```python
from build123d import *

# Parameters (mm, degrees)
EXTRUDE_1_DEPTH          = 3
SKETCH_13_W              = 40
SKETCH_13_H              = 2
EXTRUDE_3_DEPTH          = 15
EXTRUDE_4_DEPTH          = 20
EXTRUDE_4_DEPTH_BACK     = 20
CUT_EXTRUDE_6_DEPTH      = 18.5
CUT_EXTRUDE_6_DEPTH_BACK = 18.5
CUT_EXTRUDE_7_REACH      = 114.258
SKETCH_16_R              = 1.8
SKETCH_16_R_2            = 3.5


with BuildPart() as part:
    # 草图2 → 凸台-拉伸1 (new body)
    with BuildSketch(Plane.XY):
        with BuildLine():
            Line((0, 0), (63, 0))
            Line((63, 0), (63, 69))
            ThreePointArc((63, 69), (59.939265863, 76.389265863), (52.55, 79.45))
            Line((52.55, 79.45), (10.45, 79.45))
            ThreePointArc((10.45, 79.45), (3.060734137, 76.389265863), (0, 69))
            Line((0, 69), (0, 0))
        make_face()
    extrude(amount=EXTRUDE_1_DEPTH)

    # 草图13 → 凸台-拉伸3 (add)
    with BuildSketch(Plane(origin=(0, 0, 3), x_dir=(-1, 0, 0), z_dir=(0, 0, -1))):
        with Locations((-31.5, 80.45)):
            Rectangle(SKETCH_13_W, SKETCH_13_H)
    extrude(amount=EXTRUDE_3_DEPTH)

    # 草图14 → 凸台-拉伸4 (add, two sides: drawn at the far end of the back side and taken through both)
    with BuildSketch(Plane.ZY.offset(-31.5).offset(-EXTRUDE_4_DEPTH_BACK)):
        with BuildLine():
            ThreePointArc((3, 79.45), (10.588190451, 78.450995775), (16.660254038, 83.110254038))
            ThreePointArc((16.660254038, 83.110254038), (17.659258263, 85.522063587), (18, 88.110254038))
            ThreePointArc((18, 88.110254038), (11.686285655, 97.406021788), (0.717740386, 94.9636251))
            ThreePointArc((0.717740386, 94.9636251), (-1.999142036, 88.241244641), (0.540709407, 81.45))
            Line((0.540709407, 81.45), (3, 81.45))
            Line((3, 81.45), (3, 79.45))
        make_face()
        with BuildLine():
            ThreePointArc((0.540709407, 81.45), (1.690603791, 80.351934666), (3, 79.45))
            Line((3, 79.45), (3, 81.45))
            Line((3, 81.45), (0.540709407, 81.45))
        make_face()
        with BuildLine():
            ThreePointArc((0.540709407, 81.45), (-1.999142036, 88.241244641), (0.717740386, 94.9636251))
            Line((0.717740386, 94.9636251), (-12, 81.45))
            Line((-12, 81.45), (0.540709407, 81.45))
        make_face()
        with BuildLine():
            Line((3, 59.45), (16.660254038, 83.110254038))
            ThreePointArc((16.660254038, 83.110254038), (10.588190451, 78.450995775), (3, 79.45))
            Line((3, 79.45), (3, 59.45))
        make_face()
    extrude(amount=EXTRUDE_4_DEPTH + EXTRUDE_4_DEPTH_BACK)

    # 草图15 → 切除-拉伸6 (cut, two sides: drawn at the far end of the back side and taken through both)
    with BuildSketch(Plane.ZY.offset(-31.5).offset(-CUT_EXTRUDE_6_DEPTH_BACK)):
        with BuildLine():
            Line((0, 59.45), (3, 59.45))
            Line((3, 59.45), (16.660254038, 83.110254038))
            ThreePointArc((16.660254038, 83.110254038), (13.96660025, 96.13519525), (0.717740386, 94.9636251))
            Line((0.717740386, 94.9636251), (-12, 81.45))
            Line((-12, 81.45), (0, 81.45))
            Line((0, 81.45), (0, 59.45))
        make_face()
    extrude(amount=CUT_EXTRUDE_6_DEPTH + CUT_EXTRUDE_6_DEPTH_BACK, mode=Mode.SUBTRACT)

    # 切除-拉伸7: up to this face of the body (flat: up to its plane)
    cut_extrude_7_end = Plane(part.part.faces().sort_by_distance((51.5, 84.002247989, 5.535309017))[0])
    # 草图16 → 切除-拉伸7 (cut, up to the picked face)
    with BuildSketch(Plane.ZY.offset(-11.5), mode=Mode.PRIVATE) as cut_extrude_7_sk1:
        with Locations(Location((8, 95.110254038, 0), (0, 0, 270))):
            Circle(SKETCH_16_R)
    cut_extrude_7_tool1 = split(extrude(cut_extrude_7_sk1.sketch, amount=-CUT_EXTRUDE_7_REACH, mode=Mode.PRIVATE), bisect_by=cut_extrude_7_end, keep=Keep.BOTH, mode=Mode.PRIVATE)
    # 草图16 → 切除-拉伸7 (cut, up to the picked face)
    with BuildSketch(Plane.ZY.offset(-11.5), mode=Mode.PRIVATE) as cut_extrude_7_sk2:
        with Locations(Location((15, 88.110254038, 0), (0, 0, 270))):
            Circle(SKETCH_16_R)
    cut_extrude_7_tool2 = split(extrude(cut_extrude_7_sk2.sketch, amount=-CUT_EXTRUDE_7_REACH, mode=Mode.PRIVATE), bisect_by=cut_extrude_7_end, keep=Keep.BOTH, mode=Mode.PRIVATE)
    # 草图16 → 切除-拉伸7 (cut, up to the picked face)
    with BuildSketch(Plane.ZY.offset(-11.5), mode=Mode.PRIVATE) as cut_extrude_7_sk3:
        with Locations(Location((8, 81.110254038, 0), (0, 0, 270))):
            Circle(SKETCH_16_R)
    cut_extrude_7_tool3 = split(extrude(cut_extrude_7_sk3.sketch, amount=-CUT_EXTRUDE_7_REACH, mode=Mode.PRIVATE), bisect_by=cut_extrude_7_end, keep=Keep.BOTH, mode=Mode.PRIVATE)
    # 草图16 → 切除-拉伸7 (cut, up to the picked face)
    with BuildSketch(Plane.ZY.offset(-11.5), mode=Mode.PRIVATE) as cut_extrude_7_sk4:
        with Locations(Location((1, 88.110254038, 0), (0, 0, 270))):
            Circle(SKETCH_16_R)
    cut_extrude_7_tool4 = split(extrude(cut_extrude_7_sk4.sketch, amount=-CUT_EXTRUDE_7_REACH, mode=Mode.PRIVATE), bisect_by=cut_extrude_7_end, keep=Keep.BOTH, mode=Mode.PRIVATE)
    # 草图16 → 切除-拉伸7 (cut, up to the picked face)
    with BuildSketch(Plane.ZY.offset(-11.5), mode=Mode.PRIVATE) as cut_extrude_7_sk5:
        with Locations(Location((8, 88.110254038, 0), (0, 0, 270))):
            Circle(SKETCH_16_R_2)
    cut_extrude_7_tool5 = split(extrude(cut_extrude_7_sk5.sketch, amount=-CUT_EXTRUDE_7_REACH, mode=Mode.PRIVATE), bisect_by=cut_extrude_7_end, keep=Keep.BOTH, mode=Mode.PRIVATE)
    add(cut_extrude_7_tool1.solids().sort_by(Axis((11.5, 95.110254, 8), (1, 0, 0)))[0], mode=Mode.SUBTRACT)
    add(cut_extrude_7_tool2.solids().sort_by(Axis((11.5, 88.110254, 15), (1, 0, 0)))[0], mode=Mode.SUBTRACT)
    add(cut_extrude_7_tool3.solids().sort_by(Axis((11.5, 81.110254, 8), (1, 0, 0)))[0], mode=Mode.SUBTRACT)
    add(cut_extrude_7_tool4.solids().sort_by(Axis((11.5, 88.110254, 1), (1, 0, 0)))[0], mode=Mode.SUBTRACT)
    add(cut_extrude_7_tool5.solids().sort_by(Axis((11.5, 88.110254, 8), (1, 0, 0)))[0], mode=Mode.SUBTRACT)


solid = part.part
```
Part model, mm, in its own coordinate system. A direction names the side the tool comes from. Give positions to 0.01 mm unless a question says otherwise; leave off trailing zeros. Order: outer loops, then holes, each group sorted by start corner. A loop starts at its lowest first (then second) coordinate and runs counter-clockwise, first axis right, second up. Notation, with made-up numbers: M 8,-27 L 20,-27 A22 cw 20,-20 Z; hole C 40.25,-29.75 d10. An arc over 180 degrees is marked long. Use a Markdown table: item, result. Add a question column.
(1) Saw through at D-D, the plane z = 15. Give the cut face in (x, y), and give its area (3 significant figures).
(2) Drop flat-ended pins along their axis: P1, Ø4, axis at y = 81.11, z = 8, coming from the -X side; P2, Ø15, axis at y = 79.5, z = -3, coming from the -X side; P3, Ø1.6, axis at x = 37.5, y = 80, coming from the +Z side. Give the stop position or say it passes through.
(3) Mould opens along Y. For faces 4 (the face through (12.24, 86.448, 0.311)), 5 (the face through (63, 34, 1)), 6 (the face through (50.74, 93.448, 7.311)), 7 (the face through (50.76, 71.11, 9.73)) say: +Y half, -Y half, draft (parallel to the pull), parting line (faces both ways), or undercut.
(4) Probe line 1 along X through (y, z) = (70, 4.5); line 2 along Y through (x, z) = (18, -3.5); line 3 along Z through (x, y) = (56.5, 20.5). List the from-to ranges inside material, lowest first. Write a range as [from, to].
(5) Saw through at B-B, the plane z = 8. Give the number of separate pieces and of enclosed holes in the cut face, and give its area (3 significant figures).
(6) 3-axis set-ups, long thin cutter, end or side, ignore diameter. For faces 1 (the face through (50.76, 88.301, -5.552)), 2 (the face through (32, 59.45, 1)), 3 (the face through (32, 80, 0)): which of +Z, -Z, +X, -X, +Y, -Y reach the whole face in a straight line?
(7) Saw through at C-C, the plane y = 66.5. Give the cut face in (x, z).
(8) Saw through at A-A, the plane x = 26.5. Give the cut face in (y, z).
Answer key:
| question | item | result |
|---|---|---|
| 1 | outline | M 11.5,80.23 L 13,80.23 L 13,86.31 L 11.5,86.31 Z; M 11.5,89.91 L 13,89.91 L 13,95.25 L 11.5,95.25 Z; M 50,80.23 L 51.5,80.23 L 51.5,86.31 L 50,86.31 Z; M 50,89.91 L 51.5,89.91 L 51.5,95.25 L 50,95.25 Z |
| 1 | area | 34.3 mm^2 |
| 2 | P1 | x = 11.5 |
| 2 | P2 | x = 0.65 |
| 2 | P3 | z = 0 |
| 3 | face 4 | undercut |
| 3 | face 5 | draft |
| 3 | face 6 | undercut |
| 3 | face 7 | -Y half |
| 4 | line 1 | [11.5, 13], [50, 51.5] |
| 4 | line 2 | [79.45, 81.45] |
| 4 | line 3 | [0, 3] |
| 5 | separate pieces | 8 |
| 5 | enclosed holes | 0 |
| 5 | area | 47.4 mm^2 |
| 6 | face 1 | -Z, +X, -X, +Y |
| 6 | face 2 | +Z, -Z, +Y |
| 6 | face 3 | +Z, +Y |
| 7 | outline | M 0,0 L 13,0 L 13,7.07 L 11.5,7.07 L 11.5,3 L 0,3 Z; M 50,0 L 63,0 L 63,3 L 51.5,3 L 51.5,7.07 L 50,7.07 Z |
| 8 | outline | M 0,0 L 59.45,0 L 59.45,3 L 0,3 Z; M 79.45,-12 L 81.45,-12 L 81.45,0 L 79.45,0 Z |
